Autodesk Inventor part; units mm, degrees
ref_plane "YZ Plane" through (0, 0, 0) normal (1, 0, 0) x (0, 1, 0)
ref_plane "XZ Plane" through (0, 0, 0) normal (0, 1, 0) x (-1, 0, 0)
ref_plane "XY Plane" through (0, 0, 0) normal (0, 0, 1) x (1, 0, 0)
sketch "Sketch1" plane through (0, 0, 0) normal (0, 0, 1) x (1, 0, 0)
  line L0 (-21.15, -21.15) -> (21.15, -21.15)
  line L1 (21.15, -21.15) -> (21.15, 21.15)
  line L2 (21.15, 21.15) -> (-21.15, 21.15)
  line L3 (-21.15, 21.15) -> (-21.15, -21.15)
  line L4 (-21.15, -21.15) -> (21.15, 21.15) construction
  line L5 (21.15, -21.15) -> (-21.15, 21.15) construction
  point P0 (0, 0)
  dimension "d0" = 42.3
  dimension "d1" = 42.3
extrude "Extrusion1" add sketch "Sketch1" along normal blind 40
chamfer "Chamfer1" distance 5 angle 45 4 edges at (21.15, -21.15, 20) (-21.15, -21.15, 20) (21.15, 21.15, 20) (-21.15, 21.15, 20)
sketch "Sketch2" plane through (0, 0, 40) normal (0, 0, 1) x (1, 0, 0)
  circle A0 centre (0, 0) radius 18
  dimension "d7" = 36
extrude "Extrusion2" add sketch "Sketch2" along normal blind 35
sketch "Sketch3" plane through (0, 0, 40) normal (0, 0, 1) x (1, 0, 0)
  circle A0 centre (0, 0) radius 18
  line L0 (-21.15, 16.15) -> (-16.15, 21.15)
  line L1 (-21.15, 16.15) -> (-21.15, -16.15)
  line L2 (-16.15, -21.15) -> (-21.15, -16.15)
  line L3 (-16.15, -21.15) -> (16.15, -21.15)
  line L4 (21.15, -16.15) -> (16.15, -21.15)
  line L5 (21.15, -16.15) -> (21.15, 16.15)
  line L6 (16.15, 21.15) -> (21.15, 16.15)
  line L7 (16.15, 21.15) -> (-16.15, 21.15)
  line L8 (-15.7358, 20.15) -> (-20.15, 15.7358)
  line L9 (-20.15, 15.7358) -> (-20.15, -15.7358)
  line L10 (-20.15, -15.7358) -> (-15.7358, -20.15)
  line L11 (-15.7358, -20.15) -> (15.7358, -20.15)
  line L12 (15.7358, -20.15) -> (20.15, -15.7358)
  line L13 (20.15, -15.7358) -> (20.15, 15.7358)
  line L14 (20.15, 15.7358) -> (15.7358, 20.15)
  line L15 (15.7358, 20.15) -> (-15.7358, 20.15)
  dimension "d10" = 1
extrude "Extrusion3" add sketch "Sketch3" along normal blind 5 contours L15 L14 L13 L12 L11 L10 L9 L8
sketch "Sketch4" plane through (0, 0, 45) normal (0, 0, 1) x (1, 0, 0)
  line L0 (-15.5, -15.5) -> (15.5, -15.5) construction
  line L1 (15.5, -15.5) -> (15.5, 15.5) construction
  line L2 (15.5, 15.5) -> (-15.5, 15.5) construction
  line L3 (-15.5, 15.5) -> (-15.5, -15.5) construction
  line L4 (-15.5, -15.5) -> (15.5, 15.5) construction
  line L5 (15.5, -15.5) -> (-15.5, 15.5) construction
  point P0 (0, 0)
  dimension "d13" = 31
  dimension "d14" = 31
hole "Hole1" at (-15.5, 15.5, 45) at (15.5, 15.5, 45) at (-15.5, -15.5, 45) at (15.5, -15.5, 45) direction (0, 0, -1) diameter 5 depth 0.5
sketch "Sketch5" plane through (0, 0, 75) normal (0, 0, 1) x (1, 0, 0)
  circle A0 centre (0, 0) radius 11
  dimension "d22" = 22
extrude "Extrusion4" add sketch "Sketch5" along normal blind 2
sketch "Sketch6" plane through (0, 0, 77) normal (0, 0, 1) x (1, 0, 0)
  circle A0 centre (0, 0) radius 4
  dimension "d25" = 8
extrude "Extrusion5" add sketch "Sketch6" along normal blind 18
sketch "Sketch7" plane through (0, 0, 95) normal (0, 0, 1) x (1, 0, 0)
  line L0 (-2.6458, 4) -> (2.6458, 4)
  line L1 (2.6458, 4) -> (2.6458, 3)
  line L2 (2.6458, 3) -> (-2.6458, 3)
  line L3 (-2.6458, 3) -> (-2.6458, 4)
  circle A0 centre (0, 0) radius 4
  line L4 (0, 0) -> (0, 4)
  circle A1 centre (0, 0) radius 4
  point P0 (0, 3)
  dimension "d28" = 7
extrude "Extrusion6" cut sketch "Sketch7" against normal blind 15 contours L0 A0 L3 | L0 L1 A0 | L4 L2 A0 | A0 L2 L4
chamfer "Chamfer2" distance 0.5 angle 45 2 edges at (3.6458, 1.6458, 95) (-1.6458, -3.6458, 95)
chamfer "Chamfer3" distance 1 angle 45 8 edges at (0, 21.15, 0) (18.65, 18.65, 0) (21.15, 0, 0) (-21.15, 0, 0) (-18.65, 18.65, 0) (18.65, -18.65, 0) (0, -21.15, 0) (-18.65, -18.65, 0)
properties part number "motor con reductora"
CAD build for the part. Positions are in the model's coordinates, mm. A direction names the side the tool comes from. Give positions to 0.01 mm unless a question says otherwise; leave off trailing zeros. Loops run counter-clockwise (first coordinate to the right, second up) from the corner with the lowest first, then second, coordinate; pieces in that order, holes last. Notation, with made-up numbers: M -36.75,39.25 L 3.25,39.25 A11 ccw 3.25,47.25 Z; hole C 32,44 d8. An arc over 180 degrees is marked long. Answer in a Markdown table with one row per item. Add a question column.
Item 1: Tool access for faces 1 (the face through (17.912, -17.974, 42.465)), 2 (the face through (-20.5, 0.1, 40)), 3 (the face through (0, 20.15, 42)), 4 (the face through (-17.912, 17.974, 42.465)): list every direction of +Z, -Z, +X, -X, +Y, -Y with a clear straight run to the whole face (end or side of a thin tool).
Item 2: Band-saw the part on B-B on x = -8.5. Give the cut face in (y, z), then the cut area to 3 significant figures.
Item 3: Probe probe 1 along X at (y, z) = (-15.5, 44.7); probe 2 along Z at (x, y) = (15.5, 15). List the from-to ranges inside material, lowest first.
Item 4: Band-saw the part on C-C on y = -8. Give the cut face in (x, z).
Item 5: Drop flat-ended pins along their axis: P1, Ø2.5, axis at x = 16.5, y = 14.5, coming from the +Z side; P2, Ø4, axis at y = -5.5, z = 67.5, coming from the +X side; P3, Ø4, axis at y = 4.5, z = 43.5, coming from the -X side. Give the stop position or say it passes through.
Item 6: Band-saw the part on D-D on y = -14. Give the cut face in (x, z), then the cut area to 3 significant figures.
Item 7: Mould opens along X. For faces 5 (the face through (18.6, -18.7, 20.2)), 6 (the face through (-2.343, -17.847, 59.79)), 7 (the face through (-16, 16, 44.5)) say: +X half, -X half, draft (parallel to the pull), parting line (faces both ways), or undercut.
Item 8: Band-saw the part on A-A on y = 0. Give the cut face in (x, z).
Reply:
| question | item | result |
|---|---|---|
| 1 | face 1 | +Z, +X, -Y |
| 1 | face 2 | +Z |
| 1 | face 3 | +Z, +X, -X, +Y |
| 1 | face 4 | +Z, -X, +Y |
| 2 | outline | M -21.15,1 L -20.15,0 L 20.15,0 L 21.15,1 L 21.15,40 L 20.15,40 L 20.15,45 L 15.87,45 L 15.87,75 L 6.98,75 L 6.98,77 L -6.98,77 L -6.98,75 L -15.87,75 L -15.87,45 L -20.15,45 L -20.15,40 L -21.15,40 Z |
| 2 | area | 2,870 mm^2 |
| 3 | probe 1 | x = -20.15 to -18, -13 to 13, 18 to 20.15 |
| 3 | probe 2 | z = 0 to 44.5 |
| 4 | outline | M -21.15,1 L -20.15,0 L 20.15,0 L 21.15,1 L 21.15,40 L 20.15,40 L 20.15,45 L 16.12,45 L 16.12,75 L 7.55,75 L 7.55,77 L -7.55,77 L -7.55,75 L -16.12,75 L -16.12,45 L -20.15,45 L -20.15,40 L -21.15,40 Z |
| 5 | P1 | stops at z = 45 |
| 5 | P2 | stops at x = 17.66 |
| 5 | P3 | stops at x = -20.15 |
| 6 | outline | M -21.15,1 L -20.15,0 L 20.15,0 L 21.15,1 L 21.15,40 L 20.15,40 L 20.15,45 L 17.5,45 L 17.5,44.5 L 13.5,44.5 L 13.5,45 L 11.31,45 L 11.31,75 L -11.31,75 L -11.31,45 L -13.5,45 L -13.5,44.5 L -17.5,44.5 L -17.5,45 L -20.15,45 L -20.15,40 L -21.15,40 Z |
| 6 | area | 2,570 mm^2 |
| 7 | face 5 | +X half |
| 7 | face 6 | parting line |
| 7 | face 7 | undercut |
| 8 | outline | M -21.15,1 L -20.15,0 L 20.15,0 L 21.15,1 L 21.15,40 L 20.15,40 L 20.15,45 L 18,45 L 18,75 L 11,75 L 11,77 L 4,77 L 4,94.5 L 3.5,95 L -3.5,95 L -4,94.5 L -4,77 L -11,77 L -11,75 L -18,75 L -18,45 L -20.15,45 L -20.15,40 L -21.15,40 Z |
